Geometry: see drawing. Coordinates: mm, zero at the bounding-box minimum. A direction names the side the tool comes from. Coordinates: 2 decimals unless noted, no trailing zeros. Order: outer loops, then holes, each group sorted by start corner. A loop starts at its lowest first (then second) coordinate and runs counter-clockwise, first axis right, second up.
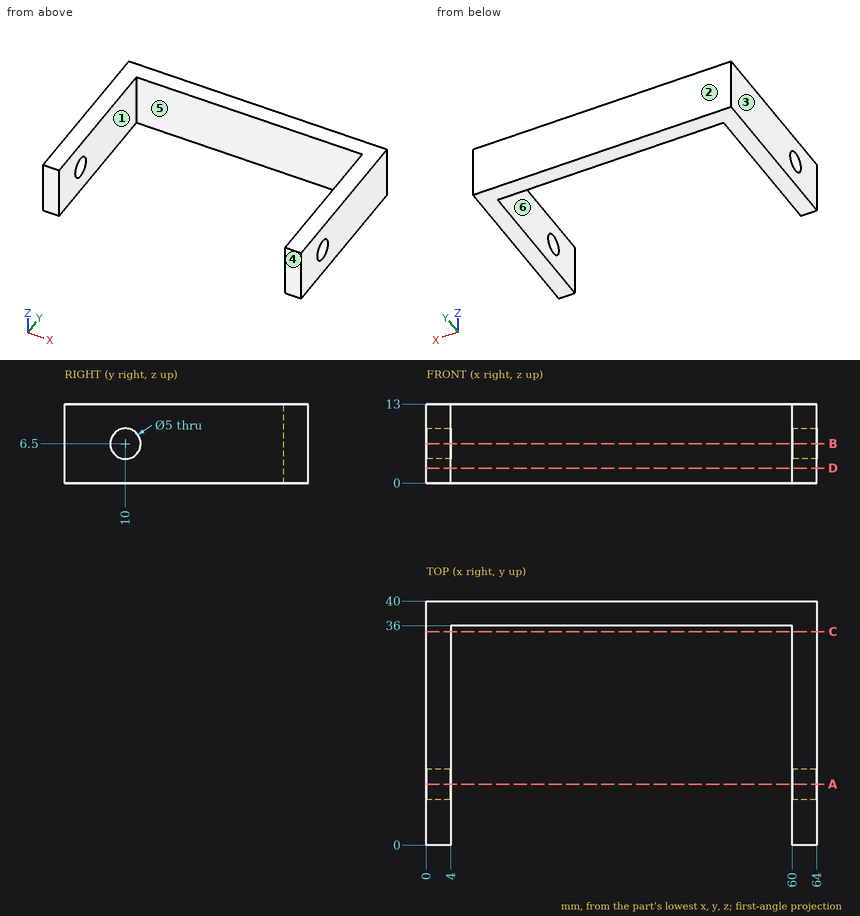
Q1. Set-up query: the marked faces 1 and 2. Return all of +Z, -Z, +X, -X, +Y, -Y with unobstructed straight access to the full face (end or side cutting, diameter ignored); none if empty.
Solutions:
face 1: +Z, -Z, -Y
face 2: +Z, -Z, +X, -X, +Y
Q2. Pull-direction query (X, two-part tool) for the marked faces 3, 4, 5 and 6; classes: pulls with the +X half, pulls with the -X half, needs draft (parallel to the pull), parting line crosses it, or undercut.
Solutions:
face 3: pulls with the -X half
face 4: needs draft
face 5: undercut
face 6: undercut
Q3. Section query C-C on y = 35. Output: boundary loops of the cut face in (x, z), plus the area to 3 significant figures.
Solutions:
outline: (0, 0) - (4, 0) - (4, 13) - (0, 13) - close; (60, 0) - (64, 0) - (64, 13) - (60, 13) - close
area: 104 mm2
Q4. Section query B-B on z = 6.5. Output: boundary loops of the cut face in (x, y), plus the area to 3 significant figures.
Solutions:
outline: (0, 0) - (4, 0) - (4, 7.5) - (0, 7.5) - close; (0, 12.5) - (4, 12.5) - (4, 36) - (60, 36) - (60, 12.5) - (64, 12.5) - (64, 40) - (0, 40) - close; (60, 0) - (64, 0) - (64, 7.5) - (60, 7.5) - close
area: 504 mm2
Q5. Section query A-A on y = 10. Output: boundary loops of the cut face in (x, z).
Solutions:
outline: (0, 0) - (4, 0) - (4, 4) - (0, 4) - close; (0, 9) - (4, 9) - (4, 13) - (0, 13) - close; (60, 0) - (64, 0) - (64, 4) - (60, 4) - close; (60, 9) - (64, 9) - (64, 13) - (60, 13) - close
Q6. Material intervals for line 1 along X through (y, z) = (19, 10.25); line 2 along Y through (x, z) = (63.05, 6.5); line 3 along Y through (x, z) = (15, 1.25), sorted ascending.
Solutions:
line 1: x = 0 to 4, 60 to 64
line 2: y = 0 to 7.5, 12.5 to 40
line 3: y = 36 to 40
Q7. Pin query (flat end, axial travel): P1, Ø3, axis at y = 18.5, z = 7.5, coming from the -X side; P2, Ø1, axis at x = 11, z = 10.5, coming from the -Y side; P3, Ø4, axis at y = 10, z = 6.5, coming from the -X side. Return the tip coordinate at first contact, or that it passes through.
Solutions:
P1: stops at x = 0
P2: stops at y = 36
P3: passes through
Q8. Section query D-D on z = 2.5. Output: boundary loops of the cut face in (x, y), plus the area to 3 significant figures.
Solutions:
outline: (0, 0) - (4, 0) - (4, 36) - (60, 36) - (60, 0) - (64, 0) - (64, 40) - (0, 40) - close
area: 544 mm2
